For this review, take the finished solid that the model builds, in its own axes (mm). Face numbers are marked on the shaded views. A direction names the side the tool comes from. Coordinates: 2 decimals unless noted, no trailing zeros. Loops run counter-clockwise (first coordinate to the right, second up) from the corner with the lowest first, then second, coordinate; pieces in that order, holes last. Notation, with made-up numbers: (16.5, 45) - (44.5, 45) arc R32 cw to (44.5, 72) - close; hole circle Ø9 at (4.25, -13.5). An arc over 180 degrees is marked (long way). Answer as a JSON object with one key per item and string values. Group by question number.
Item 1: We need section A-A (z = -13.5). Give the boundary of the cut face in (x, y), then the cut area to 3 significant figures.
Item 2: We need section C-C (x = 9.5). Give the boundary of the cut face in (y, z).
Item 3: We need section B-B (x = 20). Give the boundary of the cut face in (y, z).
Item 4: Tool access review of the marked faces 1 and 2: name each direction out of +Z, -Z, +X, -X, +Y, -Y from which nothing blocks a thin tool from reaching the whole face with its end or side.
Item 5: We need section D-D (z = -2.25). Give the boundary of the cut face in (x, y), then the cut area to 3 significant figures.
Item 6: Clearance check with flat-ended pins moving along their axes: pin 1 (1 mm diameter, centred on y = 7.5, z = -13, fed in from +X); pin 2 (5 mm diameter, centred on y = 5, z = -6.5, fed in from +X); pin 3 (10 mm diameter, centred on x = 21, z = -12.5, fed in from +Y). State where each tip first meets the part, or that it passes through.
Item 7: To check wall thickness, follow line 1 (X direction, y = 0.65, z = -10); line 2 (Y direction, x = 10, z = -16.5); line 3 (X direction, y = 0.4, z = -13.5). State the ranges of each line that lie inside material, in increasing order.
from build123d import *

# Parameters (mm, degrees)
SKETCH1_W           = 48
SKETCH1_H           = 20
SKETCH1_R           = 1.5
BOSS_EXTRUDE1_DEPTH = 1.6
SKETCH2_R           = 2.719189152
BOSS_EXTRUDE2_DEPTH = 7.5


with BuildPart() as part:
    # Sketch1 → Boss-Extrude1 (new body)
    with BuildSketch(Plane(origin=(0, 0, 0), x_dir=(1, 0, 0), z_dir=(0, 1, 0))):
        with Locations((24, 10)):
            Rectangle(SKETCH1_W, SKETCH1_H)
        with Locations(Location((20, 10, 0), (0, 0, 270))):
            Circle(SKETCH1_R, mode=Mode.SUBTRACT)
        with Locations(Location((38, 13.5, 0), (0, 0, 270))):
            Circle(SKETCH1_R, mode=Mode.SUBTRACT)
    extrude(amount=BOSS_EXTRUDE1_DEPTH)

    # Sketch2 → Boss-Extrude2 (add)
    with BuildSketch(Plane(origin=(0, 1.6, 0), x_dir=(1, 0, 0), z_dir=(0, 1, 0))):
        with Locations(Location((41.98482637, 8.947145481, 0), (0, 0, 90))):
            Circle(SKETCH2_R)
    extrude(amount=BOSS_EXTRUDE2_DEPTH)


solid = part.part
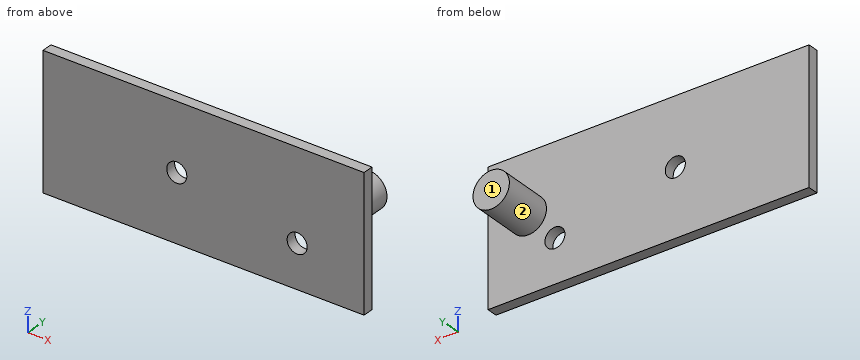
Check sheet entries:
{
 "1": {"outline": "(0, 0) - (36.5, 0) - (36.5, 1.6) - (0, 1.6) - close; (39.5, 0) - (48, 0) - (48, 1.6) - (39.5, 1.6) - close", "area": "72.0 mm2"},
 "2": {"outline": "(0, -20) - (1.6, -20) - (1.6, 0) - (0, 0) - close"},
 "3": {"outline": "(0, -20) - (1.6, -20) - (1.6, -11.5) - (0, -11.5) - close; (0, -8.5) - (1.6, -8.5) - (1.6, 0) - (0, 0) - close"},
 "4": {"face 1": "+Z, -Z, +X, -X, +Y", "face 2": "+Y"},
 "5": {"outline": "(0, 0) - (48, 0) - (48, 1.6) - (0, 1.6) - close", "area": "76.8 mm2"},
 "6": {"pin 1": "passes through", "pin 2": "stops at x = 44.7", "pin 3": "stops at y = 1.6"},
 "7": {"line 1": "x = 0 to 18.5, 21.5 to 48", "line 2": "y = 0 to 1.6", "line 3": "x = 0 to 36.5, 39.5 to 48"}
}
